Design review of the part shown in the three views and the two pictorial views. Dimensions are in mm from the part's minimum x, y and z. Give positions to 0.01 mm unless a question says otherwise; leave off trailing zeros. Order: outer loops, then holes, each group sorted by start corner. A loop starts at its lowest first (then second) coordinate and runs counter-clockwise, first axis right, second up.
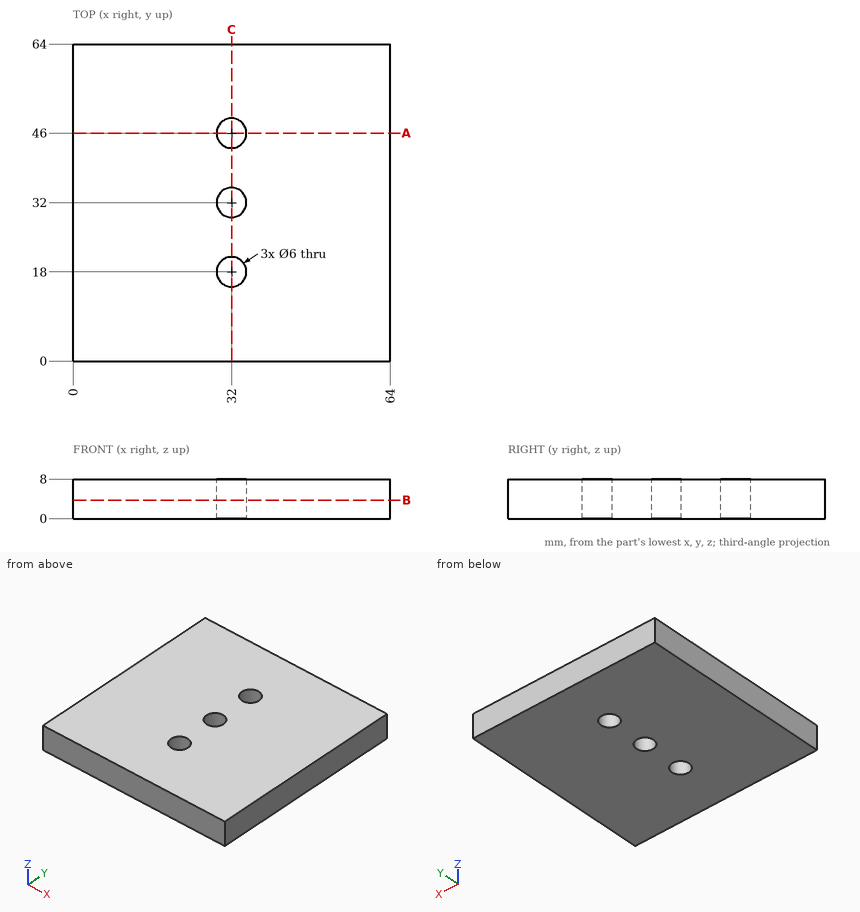
1) We need section B-B on z = 3.75. Give the boundary of the cut face in (x, y), then the cut area to 3 significant figures.
Answer sheet:
outline: (0, 0) - (64, 0) - (64, 64) - (0, 64) - close; hole circle Ø6 at (32, 18); hole circle Ø6 at (32, 32); hole circle Ø6 at (32, 46)
area: 4,010 mm2
2) We need section A-A on y = 46. Give the boundary of the cut face in (x, z).
Answer sheet:
outline: (0, 0) - (29, 0) - (29, 8) - (0, 8) - close; (35, 0) - (64, 0) - (64, 8) - (35, 8) - close
3) We need section C-C on x = 32. Give the boundary of the cut face in (y, z), then the cut area to 3 significant figures.
Answer sheet:
outline: (0, 0) - (15, 0) - (15, 8) - (0, 8) - close; (21, 0) - (29, 0) - (29, 8) - (21, 8) - close; (35, 0) - (43, 0) - (43, 8) - (35, 8) - close; (49, 0) - (64, 0) - (64, 8) - (49, 8) - close
area: 368 mm2
4) To check wall thickness, follow line 1 (Y direction, x = 32, z = 5.25); line 2 (X direction, y = 18, z = 4.75). State the ranges of each line that lie inside material, in increasing order.
Answer sheet:
line 1: y = 0 to 15, 21 to 29, 35 to 43, 49 to 64
line 2: x = 0 to 29, 35 to 64
